```python
from build123d import *

# Parameters (mm, degrees)
SKETCH1_W           = 464
SKETCH1_H           = 512
BOSS_EXTRUDE1_DEPTH = 2
SKETCH2_R           = 10
CUT_EXTRUDE1_DEPTH  = 10
SKETCH3_R           = 2.15
CUT_EXTRUDE2_DEPTH  = 10
SKETCH4_R           = 3.15
CUT_EXTRUDE3_DEPTH  = 10


with BuildPart() as part:
    # Sketch1 → Boss-Extrude1 (new body)
    with BuildSketch(Plane(origin=(0, 0, 0), x_dir=(1, 0, 0), z_dir=(0, 1, 0))):
        Rectangle(SKETCH1_W, SKETCH1_H)
    extrude(amount=BOSS_EXTRUDE1_DEPTH)

    # Sketch2 → Cut-Extrude1 (cut)
    with BuildSketch(Plane(origin=(0, 2, 0), x_dir=(1, 0, 0), z_dir=(0, 1, 0))):
        with Locations(Location((0, 0, 0), (0, 0, 270))):
            Circle(SKETCH2_R)
    extrude(amount=-CUT_EXTRUDE1_DEPTH, mode=Mode.SUBTRACT)

    # Sketch3 → Cut-Extrude2 (cut)
    with BuildSketch(Plane(origin=(0, 2, 0), x_dir=(1, 0, 0), z_dir=(0, 1, 0))):
        with Locations(Location((-10.25, 51, 0), (0, 0, 270))):
            Circle(SKETCH3_R)
        with Locations(Location((-10.25, 35, 0), (0, 0, 270))):
            Circle(SKETCH3_R)
        with Locations(Location((10.25, 35, 0), (0, 0, 90))):
            Circle(SKETCH3_R)
        with Locations(Location((10.25, 51, 0), (0, 0, 90))):
            Circle(SKETCH3_R)
        with Locations(Location((35, 10.25, 0), (0, 0, 270))):
            Circle(SKETCH3_R)
        with Locations(Location((51, 10.25, 0), (0, 0, 270))):
            Circle(SKETCH3_R)
        with Locations(Location((51, -10.25, 0), (0, 0, 90))):
            Circle(SKETCH3_R)
        with Locations(Location((35, -10.25, 0), (0, 0, 90))):
            Circle(SKETCH3_R)
        with Locations(Location((10.25, -35, 0), (0, 0, 270))):
            Circle(SKETCH3_R)
        with Locations(Location((10.25, -51, 0), (0, 0, 270))):
            Circle(SKETCH3_R)
        with Locations(Location((-10.25, -51, 0), (0, 0, 90))):
            Circle(SKETCH3_R)
        with Locations(Location((-10.25, -35, 0), (0, 0, 90))):
            Circle(SKETCH3_R)
        with Locations(Location((-35, -10.25, 0), (0, 0, 270))):
            Circle(SKETCH3_R)
        with Locations(Location((-51, -10.25, 0), (0, 0, 270))):
            Circle(SKETCH3_R)
        with Locations(Location((-51, 10.25, 0), (0, 0, 90))):
            Circle(SKETCH3_R)
        with Locations(Location((-35, 10.25, 0), (0, 0, 90))):
            Circle(SKETCH3_R)
    extrude(amount=-CUT_EXTRUDE2_DEPTH, mode=Mode.SUBTRACT)

    # Sketch4 → Cut-Extrude3 (cut)
    with BuildSketch(Plane(origin=(0, 2, 0), x_dir=(1, 0, 0), z_dir=(0, 1, 0))):
        with Locations(Location((-215, -199, 0), (0, 0, 270))):
            Circle(SKETCH4_R)
        with Locations(Location((-175, -239, 0), (0, 0, 270))):
            Circle(SKETCH4_R)
        with Locations(Location((-215, 199, 0), (0, 0, 90))):
            Circle(SKETCH4_R)
        with Locations(Location((-175, 239, 0), (0, 0, 90))):
            Circle(SKETCH4_R)
        with Locations(Location((175, -239, 0), (0, 0, 90))):
            Circle(SKETCH4_R)
        with Locations(Location((215, -199, 0), (0, 0, 90))):
            Circle(SKETCH4_R)
        with Locations(Location((215, 199, 0), (0, 0, 270))):
            Circle(SKETCH4_R)
        with Locations(Location((175, 239, 0), (0, 0, 270))):
            Circle(SKETCH4_R)
    extrude(amount=-CUT_EXTRUDE3_DEPTH, mode=Mode.SUBTRACT)


solid = part.part
```
Could you check a few things on this model? Use its own coordinates, in mm. Give positions to 0.01 mm unless a question says otherwise; leave off trailing zeros. Write each loop counter-clockwise with the first axis right and the second up, starting at its lowest first coordinate (ties: lowest second). Pieces come first, ordered by that corner, then holes. Notation, with made-up numbers: (-39.75, 48.5) -> (-1.75, 48.5) arc R16 ccw to (-1.75, 76.5) -> close; hole circle Ø11 at (77.25, 61.5). An arc over 180 degrees is marked (long way). Write each question's results on one line, items separated by ' | '.
1. I want a section at A-A, the plane z = 0. Write out the boundary of the cut face in (x, y).
Check sheet entries:
outline: (-232, 0) -> (-10, 0) -> (-10, 2) -> (-232, 2) -> close; (10, 0) -> (232, 0) -> (232, 2) -> (10, 2) -> close
2. I need wall thicknesses on L1, parallel to X at y = 0.8, z = -199; L2, parallel to Z at x = 11, y = 1.05; L3, parallel to X at y = 1.6, z = 239. Which ranges of each line are inside material? Lowest first, please.
Check sheet entries:
L1: x = -232 to -218.15, -211.85 to 211.85, 218.15 to 232 | L2: z = -256 to -53.01, -48.99 to -37.01, -32.99 to 32.99, 37.01 to 48.99, 53.01 to 256 | L3: x = -232 to -178.15, -171.85 to 171.85, 178.15 to 232
3. Will these pins go through, and if not, where does the flat tip stop? pin 1 Ø4 at (x, z) = (-215, 199) entering from +Y; pin 2 Ø7 at (x, z) = (-175, -239) entering from -Y.
Check sheet entries:
pin 1: passes through | pin 2: stops at y = 0
4. If we mould it in two halves opening along Z, with no side actions, what happens to faces 1 (the cylindrical face through (-9.76, 1.01, -2.17)), 2 (the flat face through (48, 0, -4))? For each: released by +Z, released by -Z, zero draft, split by the parting line, or undercut.
Check sheet entries:
face 1: undercut | face 2: zero draft
